Autodesk Inventor part; units mm, degrees
ref_plane "YZ Plane" through (0, 0, 0) normal (1, 0, 0) x (0, 1, 0)
ref_plane "XZ Plane" through (0, 0, 0) normal (0, 1, 0) x (-1, 0, 0)
ref_plane "XY Plane" through (0, 0, 0) normal (0, 0, 1) x (1, 0, 0)
sketch "Sketch1" plane through (0, 0, 0) normal (0, 0, 1) x (1, 0, 0)
  line L0 (-5.3462, 7.1935) -> (14.6538, 7.1935)
  line L1 (14.6538, 7.1935) -> (14.6538, 0.1935)
  line L2 (14.6538, 0.1935) -> (-5.3462, 0.1935)
  line L3 (-5.3462, 0.1935) -> (-5.3462, 7.1935)
  dimension "d0" = 20
  dimension "d1" = 7
extrude "Extrusion1" add sketch "Sketch1" along normal blind 354
sketch "Boceto2" plane through (0, 0, 354) normal (0, 0, 1) x (1, 0, 0)
  line L0 (-5.3462, 7.1935) -> (-5.3462, 0.1935)
  line L1 (-5.3462, 0.1935) -> (-4.3462, 0.1935)
  line L2 (-5.3462, 0.1935) -> (14.6538, 0.1935)
  line L3 (-5.3462, 7.1935) -> (-4.3462, 7.1935)
  line L4 (14.6538, 7.1935) -> (-5.3462, 7.1935)
  line L5 (-4.3462, 7.1935) -> (-4.3462, 5.1935)
  line L6 (-4.3462, 0.1935) -> (-4.3462, 5.1935)
  line L7 (-4.3462, 5.1935) -> (14.6538, 5.1935)
  line L8 (14.6538, 5.1935) -> (13.6538, 5.1935)
  line L9 (13.6538, 5.1935) -> (13.6538, 0.1935)
  line L10 (-4.3462, 0.1935) -> (13.6538, 0.1935)
  point P0 (0, 0)
  dimension "d4" = 1
  dimension "d5" = 1
  dimension "d6" = 2
  dimension "d7" = 1
extrude "Extrusión2" cut sketch "Boceto2" against normal blind 364.5 contours L6 L7 L9 L2
properties part number "Soporte LED_L=354" material "Stainless Steel, Austenitic"
Geometry: final body of the model. Coordinates: model frame, mm. Coordinates: 2 decimals unless noted, no trailing zeros. Order: outer loops, then holes, each group sorted by start corner. A loop starts at its lowest first (then second) coordinate and runs counter-clockwise, first axis right, second up. Notation, with made-up numbers: (71.25, -33.5) -> (102.25, -33.5) arc R28 cw to (102.25, 0.5) -> close; hole circle Ø1 at (43.25, 4). An arc over 180 degrees is marked (long way). Write item = value, one per line.
(1) Cut plane C-C on x = 2. Return loops of the section in (y, z), plus the area to 3 significant figures.
Solved:
outline = (5.19, 0) -> (7.19, 0) -> (7.19, 354) -> (5.19, 354) -> close
area = 708 mm²
(2) Line query: line 1 (X direction, y = 2.75, z = 229.5); line 2 (Y direction, x = 1.75, z = 152). Output: solid intervals per line, ascending.
Solved:
line_1 = -5.35 to -4.35, 13.65 to 14.65
line_2 = 5.19 to 7.19
(3) Pull-direction query (X, two-part tool) for faces 1 (the flat face through (-5.346, 4, 175)), 2 (the flat face through (5, 7.194, 175)), 3 (the flat face through (5, 5.194, 179)), 4 (the flat face through (14.654, 4, 175)); classes: pulls with the +X half, pulls with the -X half, needs draft (parallel to the pull), parting line crosses it, or undercut.
Solved:
face_1 = pulls with the -X half
face_2 = needs draft
face_3 = undercut
face_4 = pulls with the +X half
(4) Cut plane B-B on z = 302. Return loops of the section in (x, y), plus the area to 3 significant figures.
Solved:
outline = (-5.35, 0.19) -> (-4.35, 0.19) -> (-4.35, 5.19) -> (13.65, 5.19) -> (13.65, 0.19) -> (14.65, 0.19) -> (14.65, 7.19) -> (-5.35, 7.19) -> close
area = 50.0 mm²
(5) Cut plane A-A on y = 2.25. Return loops of the section in (x, z).
Solved:
outline = (-5.35, 0) -> (-4.35, 0) -> (-4.35, 354) -> (-5.35, 354) -> close; (13.65, 0) -> (14.65, 0) -> (14.65, 354) -> (13.65, 354) -> close
(6) Pin query (flat end, axial travel): pin 1 Ø9 at (x, z) = (1.5, 261.5) entering from -Y. Return the tip coordinate at first contact, or that it passes through.
Solved:
pin_1 = 5.19
